Here's how the part is built. I have some questions about the finished solid (model axes, mm). Round coordinates to 2 decimals unless told otherwise and drop trailing zeros. Order: outer loops, then holes, each group sorted by start corner. A loop starts at its lowest first (then second) coordinate and runs counter-clockwise, first axis right, second up.
```python
from build123d import *

# Parameters (mm, degrees)
ESQUISSE1_R      = 1.25
EXTRUSION1_DEPTH = 1.5


with BuildPart() as part:
    # Esquisse1 → Extrusion1 (new body)
    with BuildSketch(Plane.XY):
        with BuildLine():
            Line((8.941739228, 20.249575294), (9.896691771, 22.412172853))
            ThreePointArc((9.896691771, 22.412172853), (0, -24.5), (-9.896691771, 22.412172853))
            Line((-9.896691771, 22.412172853), (-8.941739228, 20.249575294))
            ThreePointArc((-8.941739228, 20.249575294), (-9.831654076, 17.417815357), (-12.754966888, 17.93265026))
            ThreePointArc((-12.754966888, 17.93265026), (0, -19.75), (12.754966888, 17.93265026))
            ThreePointArc((12.754966888, 17.93265026), (9.831654076, 17.417815357), (8.941739228, 20.249575294))
        make_face()
        with Locations((11, 19.340695437)):
            Circle(ESQUISSE1_R, mode=Mode.SUBTRACT)
        with Locations(Location((-11, 19.340695437, 0), (0, 0, 180))):
            Circle(ESQUISSE1_R, mode=Mode.SUBTRACT)
    extrude(amount=EXTRUSION1_DEPTH)


solid = part.part
```
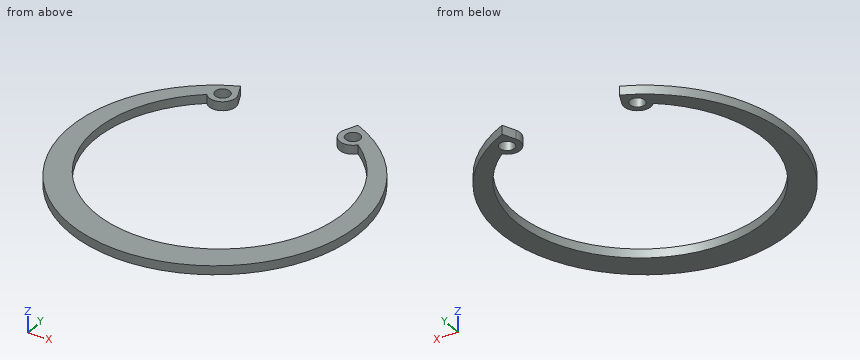
1. If we section it at A-A, the plane y = -13: Write out the boundary of the cut face in (x, z).
Evaluation:
outline: (-20.77, 0) - (-15.43, 0) - (-15.43, 1.5) - (-20.77, 1.5) - close; (15.43, 0) - (20.77, 0) - (20.77, 1.5) - (15.43, 1.5) - close
2. I'm going to push a flat-ended pin straight in: P1, Ø2, axis at x = 11, y = 19.34, coming from the -Z side. Where does the tip first touch, or does it pass through?
Evaluation:
P1: passes through
3. I need wall thicknesses on probe 1 along Y at (x, z) = (-11, 0.35); probe 2 along X at (y, z) = (19.5, 0.55); probe 3 along X at (y, z) = (1.25, 0.3). Which ranges of each line are inside material? Lowest first, please.
Evaluation:
probe 1: y = -21.89 to -16.64, 17.09 to 18.09, 20.59 to 21.89
probe 2: x = -14.83 to -12.24, -9.76 to -8.76, 8.76 to 9.76, 12.24 to 14.83
probe 3: x = -24.47 to -21, 21 to 24.47
4. If we section it at D-D, the plane x = -11: Write out the boundary of the cut face in (y, z), and give its area (3 significant figures).
Evaluation:
outline: (-21.89, 0) - (-16.64, 0) - (-16.64, 1.5) - (-21.89, 1.5) - close; (17.09, 0) - (18.09, 0) - (18.09, 1.5) - (17.09, 1.5) - close; (20.59, 0) - (21.89, 0) - (21.89, 1.5) - (20.59, 1.5) - close
area: 11.3 mm2
5. If we section it at B-B, the plane x = -17.5: Write out the boundary of the cut face in (y, z).
Evaluation:
outline: (-17.15, 0) - (-10.36, 0) - (-10.36, 1.5) - (-17.15, 1.5) - close; (12.86, 0) - (17.15, 0) - (17.15, 1.5) - (12.86, 1.5) - close
6. If we section it at C-C, the plane z = 0.8: Write out the boundary of the cut face in (x, y), and give its area (3 significant figures).
Evaluation:
outline: (-12.75, 17.93) arc R2.25 ccw to (-8.94, 20.25) - (-9.9, 22.41) arc R24.5 ccw (long way) to (9.9, 22.41) - (8.94, 20.25) arc R2.25 ccw to (12.75, 17.93) arc R21 cw (long way) to start; hole circle Ø2.5 at (-11, 19.34); hole circle Ø2.5 at (11, 19.34)
area: 460 mm2
